Autodesk Inventor part; units mm, degrees
ref_plane "YZ Plane" through (0, 0, 0) normal (1, 0, 0) x (0, 1, 0)
ref_plane "XZ Plane" through (0, 0, 0) normal (0, 1, 0) x (-1, 0, 0)
ref_plane "XY Plane" through (0, 0, 0) normal (0, 0, 1) x (1, 0, 0)
sketch "Sketch1" plane through (0, 0, 0) normal (0, 1, 0) x (-1, 0, 0)
  line L0 (0, 0) -> (-40, 0)
  line L1 (-40, 0) -> (-40, -110)
  line L2 (-40, -110) -> (0, -110)
  line L3 (0, -110) -> (0, 0)
  dimension "d0" = 110
  dimension "d1" = 40
extrude "Extrusion1" add sketch "Sketch1" along normal blind 6.5
sketch "Sketch2" plane through (0, 6.5, 0) normal (0, 1, 0) x (1, 0, 0)
  line L0 (40, 0) -> (40, 110)
  line L1 (40, 110) -> (0, 110)
  line L2 (0, 110) -> (0, 0)
  line L3 (8, 110) -> (16, 110)
  line L4 (16, 110) -> (16, 114.5)
  line L5 (14, 116.5) -> (10, 116.5)
  line L6 (8, 114.5) -> (8, 110)
  line L7 (24, 110) -> (32, 110)
  line L8 (32, 110) -> (32, 114.5)
  line L9 (30, 116.5) -> (26, 116.5)
  line L10 (24, 114.5) -> (24, 110)
  arc A0 (10, 116.5) -> (8, 114.5) centre (10, 114.5) ccw
  arc A1 (16, 114.5) -> (14, 116.5) centre (14, 114.5) ccw
  arc A2 (26, 116.5) -> (24, 114.5) centre (26, 114.5) ccw
  arc A3 (32, 114.5) -> (30, 116.5) centre (30, 114.5) ccw
  line L11 (8, 112.25) -> (0, 112.25) construction
  line L12 (16, 112.25) -> (24, 112.25) construction
  line L13 (32, 112.25) -> (40, 112.25) construction
  line L14 (0, 55) -> (40, 55) construction
  line L15 (0, 0) -> (40, 0)
  line L16 (40, 0) -> (40, 110)
  line L17 (40, 110) -> (0, 110)
  line L18 (0, 110) -> (0, 0)
  line L19 (8, 0) -> (16, 0)
  line L20 (16, 0) -> (16, -7.5)
  line L21 (14, -9.5) -> (10, -9.5)
  line L22 (8, -7.5) -> (8, 0)
  line L23 (24, 0) -> (32, 0)
  line L24 (32, 0) -> (32, -7.5)
  line L25 (30, -9.5) -> (26, -9.5)
  line L26 (24, -7.5) -> (24, 0)
  arc A4 (8, -7.5) -> (10, -9.5) centre (10, -7.5) ccw
  arc A5 (14, -9.5) -> (16, -7.5) centre (14, -7.5) ccw
  arc A6 (24, -7.5) -> (26, -9.5) centre (26, -7.5) ccw
  arc A7 (30, -9.5) -> (32, -7.5) centre (30, -7.5) ccw
  dimension "d4" = 2
  dimension "d5" = 8
  dimension "d6" = 8
  dimension "d7" = 6.5
  dimension "d10" = 2
  dimension "d11" = 9.5
extrude "Extrusion3" add sketch "Sketch2" against normal blind 6.5 contours L24 A7 L25 A6 L26 L15 | L1 L10 A2 L9 A3 L8 | L20 A5 L21 A4 L22 L15 | L1 L6 A0 L5 A1 L4
sketch "Sketch3" plane through (0, 0, 0) normal (0, -1, 0) x (1, 0, 0)
  line L0 (0, -110) -> (0, 0)
  line L1 (40, 0) -> (40, -110)
  line L2 (8, 7.5) -> (8, 0)
  line L3 (40, 0) -> (50, 0)
  line L4 (50, 0) -> (50, -15)
  line L5 (50, -15) -> (40, -25)
  line L6 (40, -85) -> (50, -95)
  line L7 (50, -95) -> (50, -110)
  line L8 (50, -110) -> (40, -110)
  line L9 (40, -85) -> (40, -110)
  line L10 (40, 0) -> (40, -25)
  dimension "d14" = 10
  dimension "d15" = 15
  dimension "d16" = 45
  dimension "d17" = 15
extrude "Extrusion4" add sketch "Sketch3" against normal blind 6.5
equation "\"d6\" = d5"
equation "\"d17\" = d15"
properties part number "spool_stand_brace_middle_a" material "Plywood, Finish"
Input: part model. Units: mm. Frame: model coordinates. A direction names the side the tool comes from. Coordinates: 2 decimals unless noted, no trailing zeros. Loops run counter-clockwise (first coordinate to the right, second up) from the corner with the lowest first, then second, coordinate; pieces in that order, holes last. Notation, with made-up numbers: (3, 30.5) -> (43, 30.5) arc R12 cw to (43, 40.5) -> close; hole circle Ø10 at (-5, 45). An arc over 180 degrees is marked (long way). Use a Markdown table: item, result.
1) Access query for faces 1 (the flat face through (16, 3, -112)), 2 (the flat face through (40, 3, -55)), 3 (the flat face through (32, 3, 4)), 4 (the flat face through (8, 3, -112)). Directions: +Z, -Z, +X, -X, +Y, -Y. A direction counts if a zero-diameter tool reaches every point of the face in a straight line with its end or side. Return the directions, or none.
Results found:
| item | result |
|---|---|
| face 1 | -Z, +Y, -Y |
| face 2 | +X, +Y, -Y |
| face 3 | +Z, +X, +Y, -Y |
| face 4 | -Z, -X, +Y, -Y |
2) Pull-direction query (Z, two-part tool) for faces 5 (the flat face through (45, 3, -90)), 6 (the flat face through (41, 3, 0)), 7 (the flat face through (32, 3, -112)), 8 (the flat face through (4, 3, -110)); classes: released by +Z, released by -Z, zero draft, split by the parting line, or undercut.
Results found:
| item | result |
|---|---|
| face 5 | undercut |
| face 6 | released by +Z |
| face 7 | zero draft |
| face 8 | released by -Z |
3) Cut plane C-C (z = -19.5). Return the cut outline in (x, y).
Results found:
| item | result |
|---|---|
| outline | (0, 0) -> (45.5, 0) -> (45.5, 6.5) -> (0, 6.5) -> close |
4) Cut plane D-D (z = -38). Return the cut outline in (x, y), then the cut area to 3 significant figures.
Results found:
| item | result |
|---|---|
| outline | (0, 0) -> (40, 0) -> (40, 6.5) -> (0, 6.5) -> close |
| area | 260 mm2 |
5) Contact query for flat-ended pins moving along their axis: pin 1 (3 mm diameter, centred on y = 5.5, z = -64.5, fed in from +X); pin 2 (1.3 mm diameter, centred on y = 3, z = -112, fed in from +X); pin 3 (2 mm diameter, centred on y = 2.5, z = 3.5, fed in from -X). Output: stop coordinate, or through.
Results found:
| item | result |
|---|---|
| pin 1 | stops at x = 40 |
| pin 2 | stops at x = 32 |
| pin 3 | stops at x = 8 |
6) Material intervals for line 1 along X through (y, z) = (5.5, 0.5); line 2 along X through (y, z) = (1, -67.5); line 3 along Z through (x, y) = (21.5, 6), sorted ascending. Write a range as from..to.
Results found:
| item | result |
|---|---|
| line 1 | x = 8..16, 24..32 |
| line 2 | x = 0..40 |
| line 3 | z = -110..0 |
7) Cut plane A-A (x = 44.5). Return the cut outline in (y, z), then the cut area to 4 significant figures.
Results found:
| item | result |
|---|---|
| outline | (0, -110) -> (6.5, -110) -> (6.5, -89.5) -> (0, -89.5) -> close; (0, -20.5) -> (6.5, -20.5) -> (6.5, 0) -> (0, 0) -> close |
| area | 266.5 mm2 |
